Geometry: final body of the model. Coordinates: model frame, mm. Give positions to 0.01 mm unless a question says otherwise; leave off trailing zeros. Write each loop counter-clockwise with the first axis right and the second up, starting at its lowest first coordinate (ties: lowest second). Pieces come first, ordered by that corner, then holes. Notation, with made-up numbers: M 8.25,65 L 32.25,65 A20 ccw 32.25,82 Z; hole C 6,36.5 d6. An arc over 180 degrees is marked long. Use one line per item in the form item = value. Start each with the question number.
Item 1: Section query A-A on x = 145. Return loops of the section in (y, z), then the cut area to 3 significant figures.
Item 2: Section query B-B on z = 3.25. Return loops of the section in (x, y).
Item 3: Material intervals for line 1 along Y through (x, z) = (145, 5); line 2 along X through (y, z) = (15.5, 1.5); line 3 along Y through (x, z) = (18, 7.5), sorted ascending. Write a range as from..to.
Item 4: Section query C-C on y = 139.5. Return loops of the section in (x, z).
Item 5: Section query D-D on y = 84.5. Return loops of the section in (x, z).
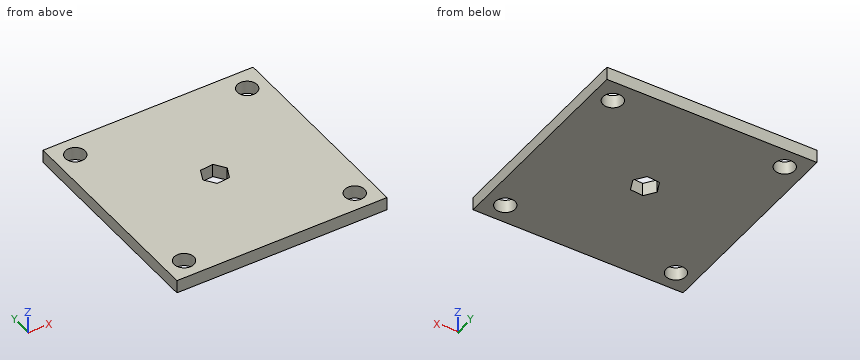
Autodesk Inventor part; units mm, degrees
ref_plane "YZ Plane" through (0, 0, 0) normal (1, 0, 0) x (0, 1, 0)
ref_plane "XZ Plane" through (0, 0, 0) normal (0, 1, 0) x (-1, 0, 0)
ref_plane "XY Plane" through (0, 0, 0) normal (0, 0, 1) x (1, 0, 0)
sketch "Sketch1" plane through (0, 0, 0) normal (0, 0, 1) x (1, 0, 0)
  line L0 (0, 0) -> (160, 0)
  line L1 (160, 0) -> (160, 160)
  line L2 (160, 160) -> (0, 160)
  line L3 (0, 160) -> (0, 0)
  dimension "d0" = 160
  dimension "d1" = 160
extrude "Extrusion1" add sketch "Sketch1" along normal blind 10
sketch "Sketch2" plane through (0, 0, 10) normal (0, 0, 1) x (1, 0, 0)
  line L0 (0, 0) -> (160, 0)
  line L1 (0, 0) -> (15, 0)
  line L2 (15, 0) -> (15, 15)
  line L3 (160, 160) -> (0, 160)
  line L4 (0, 160) -> (15, 160)
  line L5 (15, 160) -> (15, 145)
  line L6 (160, 0) -> (160, 160)
  line L7 (160, 160) -> (145, 160)
  line L8 (145, 160) -> (145, 143.5)
  line L9 (160, 0) -> (160, 15)
  line L10 (160, 15) -> (145, 15)
  circle A0 centre (15, 145) radius 7.5
  circle A1 centre (145, 143.5) radius 7.5
  circle A2 centre (145, 15) radius 7.5
  circle A3 centre (15, 15) radius 7.5
  dimension "d4" = 15
  dimension "d5" = 15
  dimension "d6" = 15
  dimension "d7" = 15
  dimension "d8" = 15
  dimension "d9" = 16.5
  dimension "d10" = 15
  dimension "d11" = 15
  dimension "d12" = 15
  dimension "d13" = 15
  dimension "d14" = 15
  dimension "d15" = 15
extrude "Extrusion2" cut sketch "Sketch2" against normal blind 10
sketch "Sketch3" plane through (0, 0, 10) normal (0, 0, 1) x (1, 0, 0)
  line L0 (0, 160) -> (0, 0)
  line L1 (0, 0) -> (80, 0)
  line L2 (0, 0) -> (160, 0)
  line L3 (80, 0) -> (0, 0)
  line L4 (0, 0) -> (80, 0)
  dimension "d18" = 80
  dimension "d19" = 80
  dimension "d20" = 80
sketch "Sketch4" plane through (0, 0, 10) normal (0, 0, 1) x (1, 0, 0)
  line L0 (0, 0) -> (160, 0)
  line L1 (0, 0) -> (0, 80)
  line L2 (0, 160) -> (0, 0)
  dimension "d21" = 80
sketch "Sketch5" plane through (0, 0, 10) normal (0, 0, 1) x (1, 0, 0)
  line L0 (0, 160) -> (0, 0)
  line L1 (0, 80) -> (80, 80)
  line L2 (84.0688, 89.1348) -> (89.9454, 81.0437)
  line L3 (89.9454, 81.0437) -> (85.8766, 71.9089)
  line L4 (85.8766, 71.9089) -> (75.9312, 70.8652)
  line L5 (75.9312, 70.8652) -> (70.0546, 78.9563)
  line L6 (70.0546, 78.9563) -> (74.1234, 88.0911)
  line L7 (74.1234, 88.0911) -> (84.0688, 89.1348)
  dimension "d22" = 80
  dimension "d23" = 10
extrude "Extrusion3" cut sketch "Sketch5" against normal blind 10
properties part number "103"
Answer sheet:
q1.outline = M 0,0 L 7.5,0 L 7.5,10 L 0,10 Z; M 22.5,0 L 136,0 L 136,10 L 22.5,10 Z; M 151,0 L 160,0 L 160,10 L 151,10 Z
q1.area = 1,300 mm2
q2.outline = M 0,0 L 160,0 L 160,160 L 0,160 Z; hole C 15,15 d15; hole C 15,145 d15; hole M 70.05,78.96 L 75.93,70.87 L 85.88,71.91 L 89.95,81.04 L 84.07,89.13 L 74.12,88.09 Z; hole C 145,15 d15; hole C 145,143.5 d15
q3.line_1 = 0..7.5, 22.5..136, 151..160
q3.line_2 = 0..7.52, 22.48..137.52, 152.48..160
q3.line_3 = 0..8.13, 21.87..138.13, 151.87..160
q4.outline = M 0,0 L 9.9,0 L 9.9,10 L 0,10 Z; M 20.1,0 L 138.66,0 L 138.66,10 L 20.1,10 Z; M 151.34,0 L 160,0 L 160,10 L 151.34,10 Z
q5.outline = M 0,0 L 72.52,0 L 72.52,10 L 0,10 Z; M 87.44,0 L 160,0 L 160,10 L 87.44,10 Z
